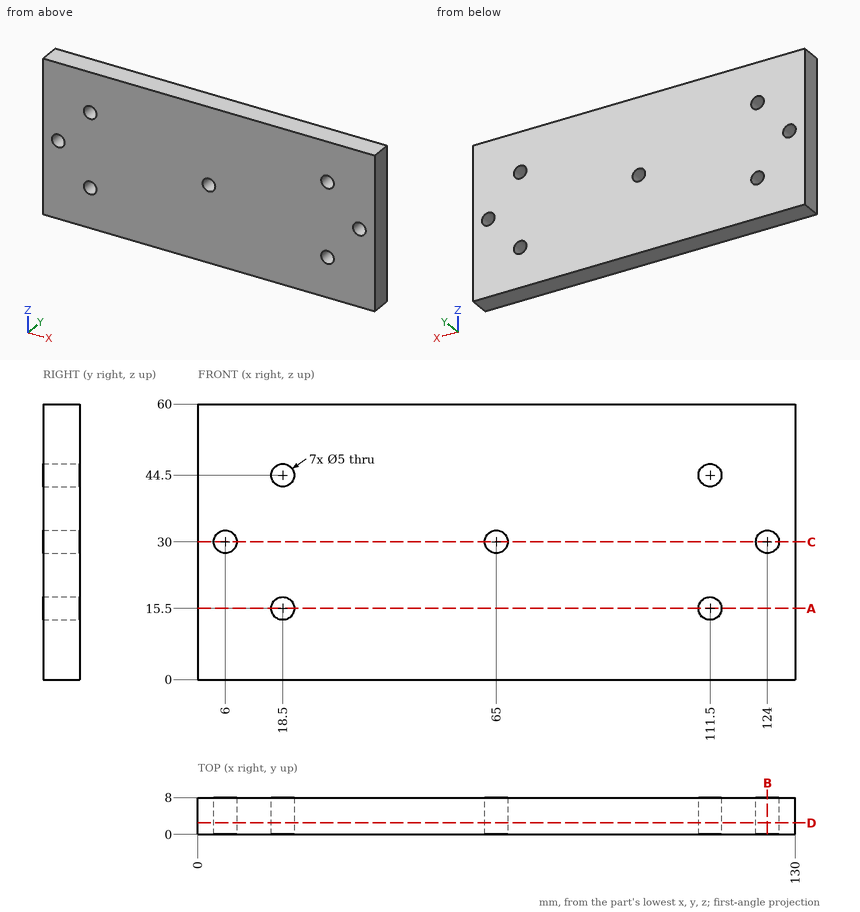
Study the drawing (mm; zero at the part's minimum x, y, z) and answer. Round coordinates to 2 decimals unless told otherwise and drop trailing zeros. Write each loop counter-clockwise with the first axis right and the second up, starting at its lowest first coordinate (ties: lowest second). Pieces come first, ordered by that corner, then holes. Notation, with made-up numbers: (18.25, 36) - (22.25, 36) arc R28 cw to (22.25, 73) - close; hole circle Ø8 at (7.25, 46.25). An arc over 180 degrees is marked (long way). Use CSV: the item, a comma, the result in double quotes.
Q1. Find section C-C, the plane z = 30. Write down the section's boundary in (x, y), then the cut area to 3 significant figures.
Values:
outline,"(0, 0) - (3.5, 0) - (3.5, 8) - (0, 8) - close; (8.5, 0) - (62.5, 0) - (62.5, 8) - (8.5, 8) - close; (67.5, 0) - (121.5, 0) - (121.5, 8) - (67.5, 8) - close; (126.5, 0) - (130, 0) - (130, 8) - (126.5, 8) - close"
area,"920 mm²"
Q2. Find section B-B, the plane x = 124. Write down the section's boundary in (y, z).
Values:
outline,"(0, 0) - (8, 0) - (8, 27.5) - (0, 27.5) - close; (0, 32.5) - (8, 32.5) - (8, 60) - (0, 60) - close"
Q3. Find section D-D, the plane y = 2.5. Write down the section's boundary in (x, z).
Values:
outline,"(0, 0) - (130, 0) - (130, 60) - (0, 60) - close; hole circle Ø5 at (6, 30); hole circle Ø5 at (18.5, 15.5); hole circle Ø5 at (18.5, 44.5); hole circle Ø5 at (65, 30); hole circle Ø5 at (111.5, 15.5); hole circle Ø5 at (111.5, 44.5); hole circle Ø5 at (124, 30)"
Q4. Straight lines are drawn through the part: line 1 along X through (y, z) = (3.75, 44.5); line 2 along X through (y, z) = (2, 30); line 3 along Z through (x, y) = (6, 2.5). For each, find the intervals that lie inside material, in ascending order.
Values:
line 1,"x = 0 to 16, 21 to 109, 114 to 130"
line 2,"x = 0 to 3.5, 8.5 to 62.5, 67.5 to 121.5, 126.5 to 130"
line 3,"z = 0 to 27.5, 32.5 to 60"
Q5. Each of these flat-tipped pins is pushed along its axis until it touches: pin 1 Ø8 at (x, z) = (6, 30) entering from -Y; pin 2 Ø3 at (x, z) = (111.5, 44.5) entering from +Y. Where does it stop, or does it pass through?
Values:
pin 1,"stops at y = 0"
pin 2,"passes through"
Q6. Find section A-A, the plane z = 15.5. Write down the section's boundary in (x, y), then the cut area to 3 significant figures.
Values:
outline,"(0, 0) - (16, 0) - (16, 8) - (0, 8) - close; (21, 0) - (109, 0) - (109, 8) - (21, 8) - close; (114, 0) - (130, 0) - (130, 8) - (114, 8) - close"
area,"960 mm²"
